```python
from build123d import *

# Parameters (mm, degrees)
SKETCH1_W           = 70
SKETCH1_H           = 35
BOSS_EXTRUDE1_DEPTH = 32
SKETCH2_R           = 4
CUT_EXTRUDE1_DEPTH  = 59.940648113
CHAMFER1_SIZE       = 25


with BuildPart() as part:
    # Sketch1 → Boss-Extrude1 (new body)
    with BuildSketch(Plane(origin=(0, 0, 0), x_dir=(1, 0, 0), z_dir=(0, 1, 0))):
        Rectangle(SKETCH1_W, SKETCH1_H)
    extrude(amount=BOSS_EXTRUDE1_DEPTH)

    # Sketch2 → Cut-Extrude1 (cut, through all)
    with BuildSketch(Plane.XY.offset(17.5)):
        with Locations((0, 25)):
            Circle(SKETCH2_R)
    extrude(amount=-CUT_EXTRUDE1_DEPTH, mode=Mode.SUBTRACT)

    # Chamfer1
    chamfer1_edges = [part.edges().sort_by_distance(p)[0] for p in [
        (-35, 32, 0),
        (35, 32, 0),
    ]]
    chamfer(chamfer1_edges, length=CHAMFER1_SIZE)


solid = part.part
```
CAD build for the part. Positions are in the model's coordinates, mm. Round coordinates to 2 decimals unless told otherwise and drop trailing zeros. Loops run counter-clockwise (first coordinate to the right, second up) from the corner with the lowest first, then second, coordinate; pieces in that order, holes last. Notation, with made-up numbers: M 88.5,2 L 137.5,2 A11 cw 137.5,21 Z; hole C 53.25,-24.75 d7. An arc over 180 degrees is marked long. Return JSON: item names as keys, results as strings. Group by question number.
(1) Saw through at B-B, the plane y = 25. List the corners of the cut face in (x, z).
(2) Saw through at A-A, the plane x = 0. List the corners of the cut face in (y, z), and give its area (3 significant figures).
(3) Wall check: probe 1 along Y at (x, z) = (0, -1); probe 2 along X at (y, z) = (23.5, 13); probe 3 along Y at (x, z) = (-21, 1.5). Give the ranges that are in metal, low to high. Write a range as [from, to].
(4) Mould opens along X. For faces 1 (the flat face through (35, 3, 0)), 2 (the cylindrical face through (-0.521, 28.966, 0.245)), 3 (the flat face through (0, 0, 0)), 4 (the flat face through (-22, 20, 0)) say: +X half, -X half, draft (parallel to the pull), parting line (faces both ways), or undercut.
(5) Saw through at D-D, the plane x = 22.5. List the corners of the cut face in (y, z).
(6) Saw through at C-C, the plane z = 7. List the corners of the cut face in (x, y), and give its area (3 significant figures).
(7) Drop flat-ended pins along their axis: P1, Ø3, axis at y = 19.5, z = -12.5, coming from the -X side; P2, Ø3, axis at y = 23, z = 2, coming from the +X side; P3, Ø1.5, axis at x = 13, z = -12, coming from the +Y side. Give the stop position or say it passes through.
Answer list:
{
 "1": {"outline": "M -17,-17.5 L -4,-17.5 L -4,17.5 L -17,17.5 Z; M 4,-17.5 L 17,-17.5 L 17,17.5 L 4,17.5 Z"},
 "2": {"outline": "M 0,-17.5 L 21,-17.5 L 21,17.5 L 0,17.5 Z; M 29,-17.5 L 32,-17.5 L 32,17.5 L 29,17.5 Z", "area": "840 mm2"},
 "3": {"probe 1": "[0, 21], [29, 32]", "probe 2": "[-18.5, -3.71], [3.71, 18.5]", "probe 3": "[0, 21]"},
 "4": {"face 1": "+X half", "face 2": "undercut", "face 3": "draft", "face 4": "-X half"},
 "5": {"outline": "M 0,-17.5 L 19.5,-17.5 L 19.5,17.5 L 0,17.5 Z"},
 "6": {"outline": "M -35,0 L 35,0 L 35,7 L 10,32 L -10,32 L -35,7 Z; hole C 0,25 d8", "area": "1,560 mm2"},
 "7": {"P1": "x = -24", "P2": "x = 20.5", "P3": "y = 29.75"}
}
